Read the model definition and answer for the solid it produces. Units are mm, in the model's axes. A direction names the side the tool comes from. Coordinates: 2 decimals unless noted, no trailing zeros. Write each loop counter-clockwise with the first axis right and the second up, starting at its lowest first coordinate (ties: lowest second). Pieces come first, ordered by that corner, then holes. Notation, with made-up numbers: (77.5, -29.75) -> (89.5, -29.75) arc R22 cw to (89.5, -5.75) -> close; hole circle Ø10 at (43, 35). An arc over 180 degrees is marked (long way). One line per item, written item: value. Start each with the question number.
1. Consider line 1 along X through (y, z) = (-13.5, 7); line 2 along X through (y, z) = (16, 5); line 3 along Y through (x, z) = (84, 8). Determine where each line is inside the solid, lowest interval first.
2. For faces 4 (the flat face through (56.709, 73, 5)), 5 (the flat face through (183.869, 44, 5)), 6 (the flat face through (171, 68.288, 5)), determine the directions among +Z, -Z, +X, -X, +Y, -Y from which every point of the face is accessible in a straight line to the end or side of a thin tool.
3. Find section C-C, the plane z = 2. State how many separate pieces and enclosed holes the cut face has, and give its area (3 significant figures).
4. Given P1, Ø5, axis at x = 73.5, z = 6.5, coming from the -Y side; P2, Ø5, axis at y = 42.5, z = 7, coming from the +X side; P3, Ø4, axis at x = 6.5, z = 5, coming from the +Y side; P4, Ø6.5, axis at x = -12.03, y = 55.59, coming from the +Z side, each flat-ended and moving along its own axis, determine where each tip first touches the part or whether it passes through.
5. Find section A-A, the plane y = -15. Write down the section's boundary in (x, z).
6. For a pull along Y with two mould halves and no side action, classify faces 1 (the flat face through (-34.731, 60, 5)), 2 (the flat face through (-30, 35.968, 5)), 3 (the flat face through (171, -12.512, 5)) as pulls with the +Y half, pulls with the -Y half, needs draft (parallel to the pull), parting line crosses it, or undercut.
7. Find section B-B, the plane x = 59. Write down the section's boundary in (y, z), and give its area (3 significant figures).
```python
from build123d import *

# Parameters (mm, degrees)
SKETCH3_R           = 4
BOSS_EXTRUDE2_DEPTH = 10


with BuildPart() as part:
    # Sketch3 → Boss-Extrude2 (new body)
    with BuildSketch(Plane.XY):
        Polygon((102.429124183, -12.51217232), (56.709124183, -12.51217232), (56.709124183, -22.51217232), (10.989124183, -22.51217232), (10.989124183, -12.51217232), (-24.730875817, -12.51217232), (-34.730875817, -12.51217232), (-34.730875817, 3.64782768), (-24.730875817, 3.64782768), (-24.730875817, 19.80782768), (-34.730875817, 19.80782768), (-34.730875817, 35.96782768), (-24.730875817, 35.96782768), (-24.730875817, 52.12782768), (-34.730875817, 52.12782768), (-34.730875817, 68.28782768), (-24.730875817, 68.28782768), (10.989124183, 68.28782768), (10.989124183, 78.28782768), (56.709124183, 78.28782768), (56.709124183, 68.28782768), (102.429124183, 68.28782768), (102.429124183, 78.28782768), (148.149124183, 78.28782768), (148.149124183, 68.28782768), (183.869124183, 68.28782768), (193.869124183, 68.28782768), (193.869124183, 52.12782768), (183.869124183, 52.12782768), (183.869124183, 35.96782768), (193.869124183, 35.96782768), (193.869124183, 19.80782768), (183.869124183, 19.80782768), (183.869124183, 3.64782768), (193.869124183, 3.64782768), (193.869124183, -12.51217232), (183.869124183, -12.51217232), (148.149124183, -12.51217232), (148.149124183, -22.51217232), (102.429124183, -22.51217232), align=None)
        with Locations((-12.030875817, 55.58782768)):
            Circle(SKETCH3_R, mode=Mode.SUBTRACT)
        with Locations((171.169124183, 55.58782768)):
            Circle(SKETCH3_R, mode=Mode.SUBTRACT)
        with Locations((-12.030875817, 0.18782768)):
            Circle(SKETCH3_R, mode=Mode.SUBTRACT)
        with Locations((171.169124183, 0.18782768)):
            Circle(SKETCH3_R, mode=Mode.SUBTRACT)
    extrude(amount=BOSS_EXTRUDE2_DEPTH)


solid = part.part
```
Answer block:
1. line 1: x = 10.99 to 56.71, 102.43 to 148.15
1. line 2: x = -24.73 to 183.87
1. line 3: y = -12.51 to 68.29
2. face 4: +Z, -Z, +Y
2. face 5: +Z, -Z, +X
2. face 6: +Z, -Z, +X, +Y
3. separate pieces: 1
3. enclosed holes: 4
3. area: 19,500 mm2
4. P1: stops at y = -12.51
4. P2: stops at x = 183.87
4. P3: stops at y = 68.29
4. P4: passes through
5. outline: (10.99, 0) -> (56.71, 0) -> (56.71, 10) -> (10.99, 10) -> close; (102.43, 0) -> (148.15, 0) -> (148.15, 10) -> (102.43, 10) -> close
6. face 1: needs draft
6. face 2: undercut
6. face 3: pulls with the -Y half
7. outline: (-12.51, 0) -> (68.29, 0) -> (68.29, 10) -> (-12.51, 10) -> close
7. area: 808 mm2
